Source: CAD feature listing. Evaluate the final solid. Frame: model axes, mm. Face numbers are marked on the shaded views. A direction names the side the tool comes from. Coordinates: 2 decimals unless noted, no trailing zeros. Order: outer loops, then holes, each group sorted by start corner. A loop starts at its lowest first (then second) coordinate and runs counter-clockwise, first axis right, second up.
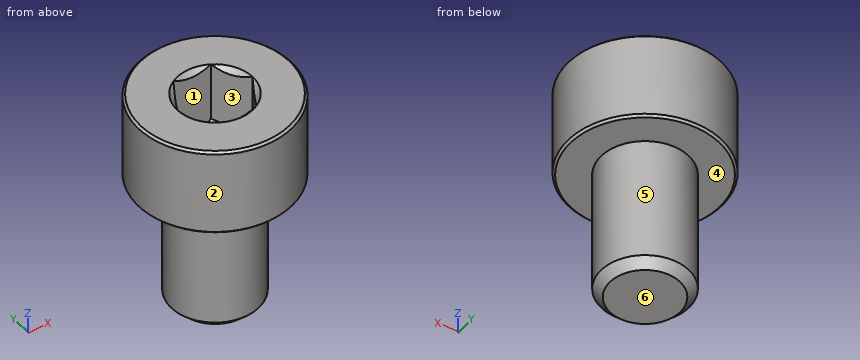
```python
from build123d import *

# Parameters (mm, degrees)
SKETCH001_R     = 3.75
POCKET_DEPTH    = 9.70192
CHAMFER_SIZE    = 0.4
CHAMFER001_SIZE = 0.1
CHAMFER002_SIZE = 0.4


with BuildPart() as pocket:
    # Sketch003 → Revolution001 (revolve)
    with BuildSketch(Plane.XZ):
        Polygon((0, 0.29908), (2.75, 1.3), (2.75, 10), (0, 10), align=None)
    revolve(axis=Axis((0, 0, 0), (0, 0, 1)))

    # Sketch001 → Pocket (cut, through all)
    with BuildSketch(Plane(origin=(0, 0, 10), x_dir=(-1, 0, 0), z_dir=(0, 0, 1))):
        Circle(SKETCH001_R)
        Polygon((-0.866025, 1.5), (0.866025, 1.5), (1.732051, 0), (0.866025, -1.5), (-0.866025, -1.5), (-1.732051, 0), align=None, mode=Mode.SUBTRACT)
    extrude(amount=-POCKET_DEPTH, mode=Mode.SUBTRACT)


with BuildPart() as chamfer002:
    # Sketch → Revolution (revolve)
    with BuildSketch(Plane.XZ):
        Polygon((1.73, 4), (3.5, 4), (3.5, 0), (2, 0), (2, -6), (0, -6), (0, 2.269998), align=None)
    revolve(axis=Axis((0, 0, 0), (0, 0, 1)))

    # Cut: cut Pocket
    add(pocket.part, mode=Mode.SUBTRACT)

    # Chamfer
    chamfer_edges = [chamfer002.edges().sort_by_distance(p)[0] for p in [
        (1.299038, 0.75, 0.845037),
    ]]
    chamfer(chamfer_edges, length=CHAMFER_SIZE)

    # Chamfer001
    chamfer001_edges = [chamfer002.edges().sort_by_distance(p)[0] for p in [
        (-3.5, 0, 4),
        (-3.5, 0, 0),
    ]]
    chamfer(chamfer001_edges, length=CHAMFER001_SIZE)

    # Chamfer002
    chamfer002_edges = [chamfer002.edges().sort_by_distance(p)[0] for p in [
        (-2, 0, -6),
    ]]
    chamfer(chamfer002_edges, length=CHAMFER002_SIZE)


solid = chamfer002.part
```
Q1. Section query B-B on z = -5. Output: boundary loops of the cut face in (x, y).
Solutions:
outline: circle Ø4 at (0, 0)
Q2. Pin query (flat end, axial travel): P1, Ø1, axis at x = -2.5, z = 2.5, coming from the -Y side; P2, Ø1, axis at x = 1, z = 2.5, coming from the -Y side; P3, Ø1, axis at x = 0.5, y = -2.5, coming from the -Z side. Return the tip coordinate at first contact, or that it passes through.
Solutions:
P1: stops at y = -2.87
P2: stops at y = -3.46
P3: stops at z = 0
Q3. Set-up query: the marked faces 5 and 6. Return all of +Z, -Z, +X, -X, +Y, -Y with unobstructed straight access to the full face (end or side cutting, diameter ignored); none if empty.
Solutions:
face 5: -Z
face 6: -Z, +X, -X, +Y, -Y
Q4. Pull-direction query (X, two-part tool) for the marked faces 1, 2, 3 and 4; classes: pulls with the +X half, pulls with the -X half, needs draft (parallel to the pull), parting line crosses it, or undercut.
Solutions:
face 1: undercut
face 2: parting line crosses it
face 3: undercut
face 4: needs draft
Q5. Material intervals for line 1 along Z through (x, y) = (2.25, -0.75); line 2 along X through (y, z) = (-0.25, 2); line 3 along Y through (x, z) = (-1, -5.25), sorted ascending.
Solutions:
line 1: z = 0 to 4
line 2: x = -3.49 to -1.59, 1.59 to 3.49
line 3: y = -1.73 to 1.73
Q6. Section query A-A on z = 2.25. Output: boundary loops of the cut face in (x, y).
Solutions:
outline: circle Ø7 at (0, 0); hole (-1.73, 0) - (-0.87, -1.5) - (0.87, -1.5) - (1.73, 0) - (0.87, 1.5) - (-0.87, 1.5) - close
